CAD build for the part. Positions are in the model's coordinates, mm. A direction names the side the tool comes from. Coordinates: 2 decimals unless noted, no trailing zeros. Loops run counter-clockwise (first coordinate to the right, second up) from the corner with the lowest first, then second, coordinate; pieces in that order, holes last. Notation, with made-up numbers: M -40,-16.75 L -29,-16.75 A8 cw -29,-11.75 Z; hole C 17,-32 d7. An arc over 180 degrees is marked long. Answer as a JSON object with one key per item and string values. Group by question number.
```python
from build123d import *

# Parameters (mm, degrees)
SKETCH1_R             = 4.7625
BOSS_EXTRUDE1_DEPTH   = 47.625
CHAMFER1_SIZE         = 1.016
CHAMFER1_SIZE2        = 0.883195326
CHAMFER1_PART_2_SIZE  = 1.016
CHAMFER1_PART_2_SIZE2 = 0.883195326
SKETCH3_W             = 0.9144
SKETCH3_H             = 0.9906


with BuildPart() as part:
    # Sketch1 → Boss-Extrude1 (new body, symmetric)
    with BuildSketch(Plane(origin=(0, 0, 0), x_dir=(1, 0, 0), z_dir=(0, 1, 0))):
        Circle(SKETCH1_R)
    extrude(amount=BOSS_EXTRUDE1_DEPTH, both=True)

    # Chamfer1
    chamfer1_edges = [part.edges().sort_by_distance(p)[0] for p in [
        (-4.7625, -47.625, 0),
    ]]
    chamfer1_side = [part.faces().sort_by_distance(p)[0] for p in [
        (0, -47.625, 0),
    ]]
    chamfer(chamfer1_edges, length=CHAMFER1_SIZE, length2=CHAMFER1_SIZE2, reference=chamfer1_side[0])

    # Chamfer1 part 2
    chamfer1_part_2_edges = [part.edges().sort_by_distance(p)[0] for p in [
        (-4.7625, 47.625, 0),
    ]]
    chamfer1_part_2_side = [part.faces().sort_by_distance(p)[0] for p in [
        (-4.7625, 0, 0),
    ]]
    chamfer(chamfer1_part_2_edges, length=CHAMFER1_PART_2_SIZE, length2=CHAMFER1_PART_2_SIZE2, reference=chamfer1_part_2_side[0])

    # Sketch3 → Cut-Revolve1 (revolve, cut)
    with BuildSketch(Plane(origin=(0, 0, 0), x_dir=(0, 0, -1), z_dir=(1, 0, 0))):
        with Locations((4.3053, 44.017653665)):
            Rectangle(SKETCH3_W, SKETCH3_H)
    revolve(axis=Axis((0, -47.820758339, 0), (0, 1, 0)), mode=Mode.SUBTRACT)


solid = part.part
```
Item 1: Pin check, flat tips, straight feed: pin 1 (1 mm diameter, centred on x = -1, y = 10.5, fed in from -Z); pin 2 (1 mm diameter, centred on x = 3, y = -4, fed in from -Z); pin 3 (5 mm diameter, centred on y = -21, z = -3.5, fed in from -X). Stop position of each tip, or through.
Item 2: Slice it at A-A, the plane y = 22. Write the cut outline in (x, z) (1 decimal), then the cut area to 3 significant figures.
Item 3: Tool access for faces 5 (the cylindrical face through (4.4, -0.98, 1.82)), 6 (the flat face through (0, 43.522, 4)): list every direction of +Z, -Z, +X, -X, +Y, -Y with a clear straight run to the whole face (end or side of a thin tool).
Item 4: Drill centre lines: L1, parallel to X at y = -20.5, z = -2.75; L2, parallel to Z at x = 0.25, y = 19; L3, parallel to Y at x = 3, z = -3.5. Where is each one in solid material? Low to high. Write a range as from..to.
Item 5: Pull direction Y, two halves, no side cores. Call faces 1 (the cylindrical face through (4.4, 45.58, 1.82)), 2 (the flat face through (0, 44.513, 4)), 3 (the flat face through (0, 47.625, 0)), 4 (the flat face through (0, -47.625, 0)): released by +Y, released by -Y, zero draft, split by the parting line, or undercut.
Computed:
{
 "1": {"pin 1": "z = -4.74", "pin 2": "z = -4.05", "pin 3": "x = -4.66"},
 "2": {"outline": "C 0,0 d9.5", "area": "71.3 mm2"},
 "3": {"face 5": "+Y, -Y", "face 6": "none"},
 "4": {"L1": "-3.89..3.89", "L2": "-4.76..4.76", "L3": "-46.87..43.52, 44.51..46.78"},
 "5": {"face 1": "zero draft", "face 2": "undercut", "face 3": "released by +Y", "face 4": "released by -Y"}
}
